```python
from build123d import *

# Parameters (mm, degrees)
SKETCH1_R           = 22
BOSS_EXTRUDE1_DEPTH = 7.7
SKETCH2_R           = 20.1
SKETCH2_R_2         = 18.1
BOSS_EXTRUDE2_DEPTH = 6.8
SKETCH3_R           = 4.15
SKETCH3_R_2         = 1.25
CUT_EXTRUDE1_DEPTH  = 15.5
SKETCH4_R           = 2.8
CUT_EXTRUDE2_DEPTH  = 3.3
SKETCH6_R           = 1.6
CUT_EXTRUDE3_DEPTH  = 15.5


with BuildPart() as part:
    # Sketch1 → Boss-Extrude1 (new body)
    with BuildSketch(Plane.XY):
        Circle(SKETCH1_R)
    extrude(amount=BOSS_EXTRUDE1_DEPTH)

    # Sketch2 → Boss-Extrude2 (add)
    with BuildSketch(Plane(origin=(0, 0, 0), x_dir=(-1, 0, 0), z_dir=(0, 0, -1))):
        Circle(SKETCH2_R)
        Circle(SKETCH2_R_2, mode=Mode.SUBTRACT)
    extrude(amount=BOSS_EXTRUDE2_DEPTH)

    # Sketch3 → Cut-Extrude1 (cut, through all)
    with BuildSketch(Plane.XY.offset(7.7)):
        Circle(SKETCH3_R)
        with Locations((0, 8)):
            Circle(SKETCH3_R_2)
        with Locations((5.656854249, 5.656854249)):
            Circle(SKETCH3_R_2)
        with Locations((8, 0)):
            Circle(SKETCH3_R_2)
        with Locations((5.656854249, -5.656854249)):
            Circle(SKETCH3_R_2)
        with Locations((0, -8)):
            Circle(SKETCH3_R_2)
        with Locations((-5.656854249, -5.656854249)):
            Circle(SKETCH3_R_2)
        with Locations((-8, 0)):
            Circle(SKETCH3_R_2)
        with Locations((-5.656854249, 5.656854249)):
            Circle(SKETCH3_R_2)
    extrude(amount=-CUT_EXTRUDE1_DEPTH, mode=Mode.SUBTRACT)

    # Sketch4 → Cut-Extrude2 (cut)
    with BuildSketch(Plane.XY.offset(7.7)):
        with Locations((14, 0)):
            Circle(SKETCH4_R)
        with Locations((0, -14)):
            Circle(SKETCH4_R)
        with Locations((-14, 0)):
            Circle(SKETCH4_R)
        with Locations((0, 14)):
            Circle(SKETCH4_R)
    extrude(amount=-CUT_EXTRUDE2_DEPTH, mode=Mode.SUBTRACT)

    # Sketch6 → Cut-Extrude3 (cut, through all)
    with BuildSketch(Plane.XY.offset(7.7)):
        with Locations((14, 0)):
            Circle(SKETCH6_R)
        with Locations((0, -14)):
            Circle(SKETCH6_R)
        with Locations((-14, 0)):
            Circle(SKETCH6_R)
        with Locations((0, 14)):
            Circle(SKETCH6_R)
    extrude(amount=-CUT_EXTRUDE3_DEPTH, mode=Mode.SUBTRACT)


solid = part.part
```
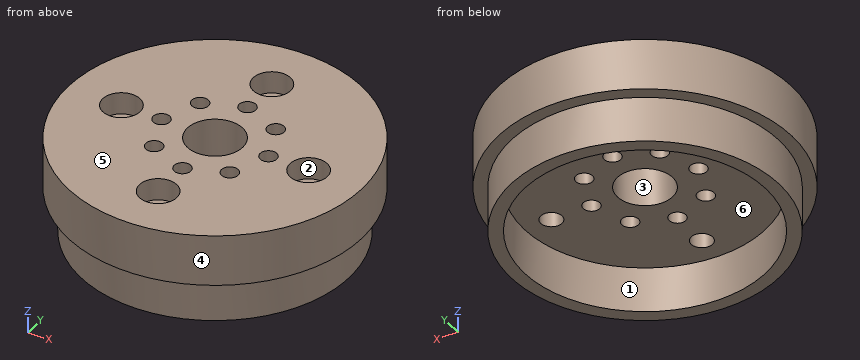
Geometry check sheet. Reference: the model listing, model coordinates, mm. Face numbers are marked on the shaded views. A direction names the side the tool comes from. Coordinates: 2 decimals unless noted, no trailing zeros. Loops run counter-clockwise (first coordinate to the right, second up) from the corner with the lowest first, then second, coordinate; pieces in that order, holes last. Notation, with made-up numbers: (83, -25) - (119, -25) arc R26 cw to (119, -2) - close; hole circle Ø9 at (15, 10). An arc over 180 degrees is marked (long way). One line per item, written item: value. Start each with the question number.
(1) Cross-section at D-D on y = -8. Enter the section's corners in (x, z).
(2) Cross-section at B-B on z = 0.75. Count the separate pieces of the cut face and the enclosed holes in it, plus the area to 3 significant figures.
(3) Tool access check on the marked faces 1, 2 and 3. Record the directions out of +Z, -Z, +X, -X, +Y, -Y that give a thin tool (end or side, any length) a straight path to the whole face; none if there is none.
(4) Mould release check, pull along Y, two halves, no side actions. Record for the marked faces 4, 5 and 6: released by +Y, released by -Y, zero draft, split by the parting line, or undercut.
(5) Cross-section at A-A on x = 5.5. Enter the section's corners in (y, z), plus the area to 3 significant figures.
(6) Depth check by flat-ended pin: P1, Ø3, axis at x = -5.66, y = 5.66, coming from the -Z side; P2, Ø1.5, axis at y = -15, z = 2, coming from the -X side; P3, Ø2, axis at y = 16, z = 5, coming from the -X side. Enter the tip coordinate at first touch or a pass-through.
(7) Cross-section at C-C on x = 14. Enter the section's corners in (y, z).
(8) Material ranges on line 1 (Z direction, x = -7, y = -15); line 2 (Y direction, x = -8, z = 3); line 3 (Y direction, x = -16.5, z = -2.75), recorded low to high. Write a range as [from, to].
Results below:
1. outline: (-20.49, 0) - (-18.44, 0) - (-18.44, -6.8) - (-16.24, -6.8) - (-16.24, 0) - (-1.25, 0) - (-1.25, 7.7) - (-20.49, 7.7) - close; (1.25, 0) - (16.24, 0) - (16.24, -6.8) - (18.44, -6.8) - (18.44, 0) - (20.49, 0) - (20.49, 7.7) - (1.25, 7.7) - close
2. separate pieces: 1
2. enclosed holes: 13
2. area: 1,390 mm2
3. face 1: -Z
3. face 2: +Z
3. face 3: +Z, -Z
4. face 4: split by the parting line
4. face 5: zero draft
4. face 6: undercut
5. outline: (-21.3, 0) - (-19.33, 0) - (-19.33, -6.8) - (-17.24, -6.8) - (-17.24, 0) - (-6.9, 0) - (-6.9, 7.7) - (-21.3, 7.7) - close; (-4.42, 0) - (4.42, 0) - (4.42, 7.7) - (-4.42, 7.7) - close; (6.9, 0) - (17.24, 0) - (17.24, -6.8) - (19.33, -6.8) - (19.33, 0) - (21.3, 0) - (21.3, 7.7) - (6.9, 7.7) - close
5. area: 318 mm2
6. P1: stops at z = 0
6. P2: stops at x = -16.76
6. P3: stops at x = -16.09
7. outline: (-16.97, 0) - (-14.42, 0) - (-14.42, -6.8) - (-11.47, -6.8) - (-11.47, 0) - (-1.6, 0) - (-1.6, 4.4) - (-2.8, 4.4) - (-2.8, 7.7) - (-16.97, 7.7) - close; (1.6, 0) - (11.47, 0) - (11.47, -6.8) - (14.42, -6.8) - (14.42, 0) - (16.97, 0) - (16.97, 7.7) - (2.8, 7.7) - (2.8, 4.4) - (1.6, 4.4) - close
8. line 1: z = [0, 7.7]
8. line 2: y = [-20.49, -1.25], [1.25, 20.49]
8. line 3: y = [-11.48, -7.44], [7.44, 11.48]
